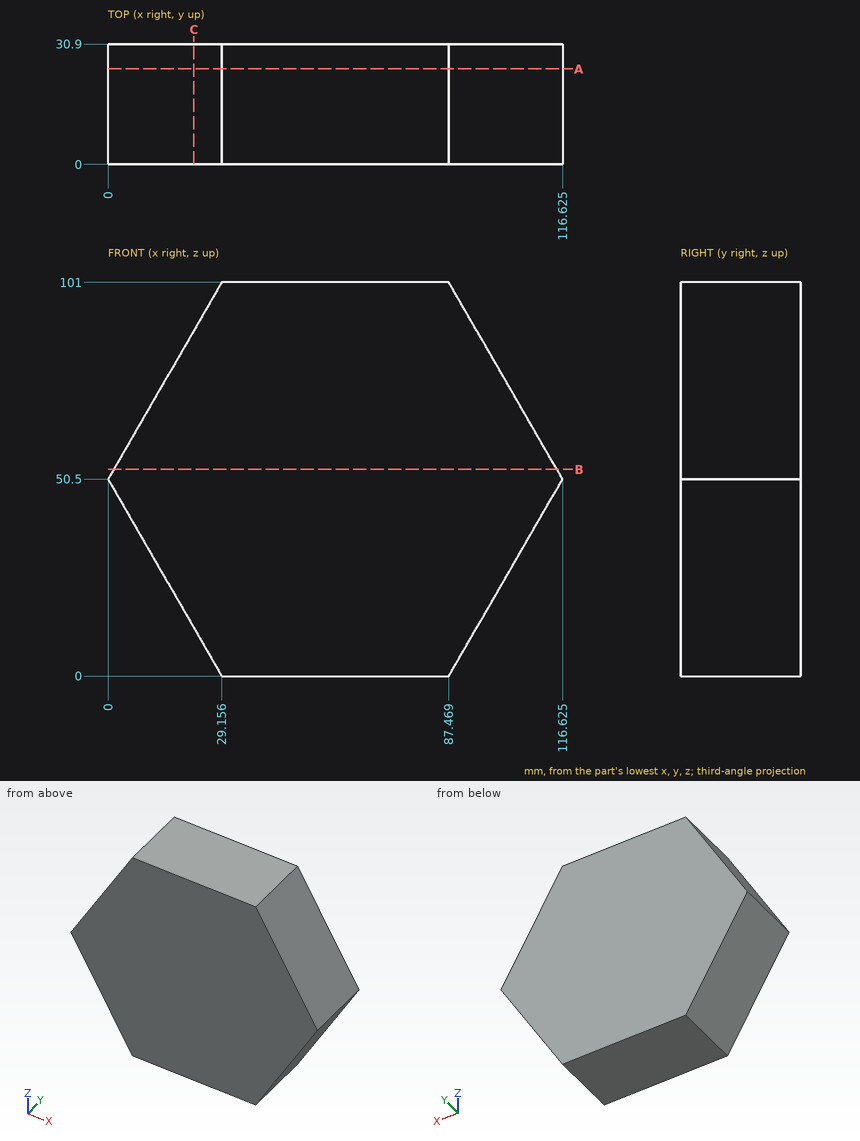
Drawing for the job (mm, zero at the part's lowest x, y, z). Round coordinates to 2 decimals unless told otherwise and drop trailing zeros. Order: outer loops, then holes, each group sorted by start corner. A loop starts at its lowest first (then second) coordinate and runs counter-clockwise, first axis right, second up. Notation, with made-up numbers: M -7.5,84 L 43.5,84 A11 ccw 43.5,100 Z; hole C -7,39.5 d10. An arc over 180 degrees is marked long. Use one line per item in the form item = value.
Q1. Flat gauge pins, fed straight in: P1, Ø12, axis at x = 33, z = 50, coming from the -Y side; P2, Ø10, axis at y = 13, z = 65, coming from the -X side (1 decimal); P3, Ø12, axis at y = 18, z = 90.5, coming from the -X side; P4, Ø2, axis at y = 22.5, z = 56, coming from the -X side. Where does each tip first touch, or does it go through?
Recorded:
P1 = 0
P2 = 5.5
P3 = 19.63
P4 = 2.6
Q2. Saw through at C-C on x = 22. Give the cut face in (y, z) (1 decimal).
Recorded:
outline = M 0,12.4 L 30.9,12.4 L 30.9,88.6 L 0,88.6 Z
Q3. Probe L1, parallel to X at y = 21, z = 58.5 (1 decimal); L2, parallel to Z at x = 95, y = 21 (1 decimal); L3, parallel to X at y = 19, z = 89. List the from-to ranges inside material, lowest first.
Recorded:
L1 = 4.6 to 112
L2 = 13 to 88
L3 = 22.23 to 94.4
Q4. Saw through at A-A on y = 24.5. Give the cut face in (x, z) (1 decimal), then the cut area to 3 significant figures.
Recorded:
outline = M 0,50.5 L 29.2,0 L 87.5,0 L 116.6,50.5 L 87.5,101 L 29.2,101 Z
area = 8,830 mm^2
Q5. Saw through at B-B on z = 53. Give the cut face in (x, y), then the cut area to 3 significant figures.
Recorded:
outline = M 1.44,0 L 115.18,0 L 115.18,30.9 L 1.44,30.9 Z
area = 3,510 mm^2
